from build123d import *

# Parameters (mm, degrees)
SKETCH1_R      = 2.5527
FINALCUT_DEPTH = 101.6


with BuildPart() as part:
    # Sketch1 → FinalCut (new body)
    with BuildSketch(Plane.XY):
        with BuildLine():
            Line((-17.4498, 0), (-17.4498, 3.187235435))
            Line((-17.4498, 3.187235435), (-23.0632, 8.800635435))
            Line((-23.0632, 8.800635435), (-23.0632, 3.2258))
            Line((-23.0632, 3.2258), (-25.4, 3.2258))
            Line((-25.4, 3.2258), (-25.4, 10.668))
            ThreePointArc((-25.4, 10.668), (-24.804840979, 12.104840979), (-23.368, 12.7))
            Line((-23.368, 12.7), (-15.9258, 12.7))
            Line((-15.9258, 12.7), (-15.9258, 10.3632))
            Line((-15.9258, 10.3632), (-21.500635435, 10.3632))
            Line((-21.500635435, 10.3632), (-15.887235435, 4.7498))
            Line((-15.887235435, 4.7498), (-12.7, 4.7498))
            Line((-12.7, 4.7498), (-9.512764565, 4.7498))
            Line((-9.512764565, 4.7498), (-3.899364565, 10.3632))
            Line((-3.899364565, 10.3632), (-9.4742, 10.3632))
            Line((-9.4742, 10.3632), (-9.4742, 12.7))
            Line((-9.4742, 12.7), (9.4742, 12.7))
            Line((9.4742, 12.7), (9.4742, 10.3632))
            Line((9.4742, 10.3632), (3.899364565, 10.3632))
            Line((3.899364565, 10.3632), (9.512764565, 4.7498))
            Line((9.512764565, 4.7498), (15.887235435, 4.7498))
            Line((15.887235435, 4.7498), (21.500635435, 10.3632))
            Line((21.500635435, 10.3632), (15.9258, 10.3632))
            Line((15.9258, 10.3632), (15.9258, 12.7))
            Line((15.9258, 12.7), (23.368, 12.7))
            ThreePointArc((23.368, 12.7), (24.804840979, 12.104840979), (25.4, 10.668))
            Line((25.4, 10.668), (25.4, 3.2258))
            Line((25.4, 3.2258), (23.0632, 3.2258))
            Line((23.0632, 3.2258), (23.0632, 8.800635435))
            Line((23.0632, 8.800635435), (17.4498, 3.187235435))
            Line((17.4498, 3.187235435), (17.4498, 0))
            Line((17.4498, 0), (17.4498, -3.187235435))
            Line((17.4498, -3.187235435), (23.0632, -8.800635435))
            Line((23.0632, -8.800635435), (23.0632, -3.2258))
            Line((23.0632, -3.2258), (25.4, -3.2258))
            Line((25.4, -3.2258), (25.4, -10.668))
            ThreePointArc((25.4, -10.668), (24.804840979, -12.104840979), (23.368, -12.7))
            Line((23.368, -12.7), (15.9258, -12.7))
            Line((15.9258, -12.7), (15.9258, -10.3632))
            Line((15.9258, -10.3632), (21.500635435, -10.3632))
            Line((21.500635435, -10.3632), (15.887235435, -4.7498))
            Line((15.887235435, -4.7498), (12.7, -4.7498))
            Line((12.7, -4.7498), (9.512764565, -4.7498))
            Line((9.512764565, -4.7498), (3.899364565, -10.3632))
            Line((3.899364565, -10.3632), (9.4742, -10.3632))
            Line((9.4742, -10.3632), (9.4742, -12.7))
            Line((9.4742, -12.7), (-9.4742, -12.7))
            Line((-9.4742, -12.7), (-9.4742, -10.3632))
            Line((-9.4742, -10.3632), (-3.899364565, -10.3632))
            Line((-3.899364565, -10.3632), (-9.512764565, -4.7498))
            Line((-9.512764565, -4.7498), (-12.7, -4.7498))
            Line((-12.7, -4.7498), (-15.887235435, -4.7498))
            Line((-15.887235435, -4.7498), (-21.500635435, -10.3632))
            Line((-21.500635435, -10.3632), (-15.9258, -10.3632))
            Line((-15.9258, -10.3632), (-15.9258, -12.7))
            Line((-15.9258, -12.7), (-23.368, -12.7))
            ThreePointArc((-23.368, -12.7), (-24.804840979, -12.104840979), (-25.4, -10.668))
            Line((-25.4, -10.668), (-25.4, -3.2258))
            Line((-25.4, -3.2258), (-23.0632, -3.2258))
            Line((-23.0632, -3.2258), (-23.0632, -8.800635435))
            Line((-23.0632, -8.800635435), (-17.4498, -3.187235435))
            Line((-17.4498, -3.187235435), (-17.4498, 0))
        make_face()
        with Locations((-12.7, 0)):
            Circle(SKETCH1_R, mode=Mode.SUBTRACT)
        with Locations(Location((12.7, 0, 0), (0, 0, 180))):
            Circle(SKETCH1_R, mode=Mode.SUBTRACT)
        Polygon((7.9502, 3.187235435), (0, 11.137435435), (-7.9502, 3.187235435), (-7.9502, 0), (-7.9502, -3.187235435), (0, -11.137435435), (7.9502, -3.187235435), (7.9502, 0), align=None, mode=Mode.SUBTRACT)
    extrude(amount=-FINALCUT_DEPTH)


solid = part.part
Work out the finished part from the listing and answer in its coordinate system (mm). A direction names the side the tool comes from. Give positions to 0.01 mm unless a question says otherwise; leave off trailing zeros. Write each loop counter-clockwise with the first axis right and the second up, starting at its lowest first coordinate (ties: lowest second). Pieces come first, ordered by that corner, then holes. Notation, with made-up numbers: (-4, -21) - (49, -21) arc R24 ccw to (49, -7) - close; hole circle Ø11 at (87, 43.5). An arc over 180 degrees is marked (long way). One line per item, written item: value. Start each with the question number.
1. Find section C-C (z = -85). State how many separate pieces and enclosed holes the cut face has, then the cut area to 3 significant figures.
2. Find section B-B (y = 0). Write down the section's boundary in (x, z), then the cut area to 3 significant figures.
3. Given pin 1 (5 mm diameter, centred on y = 3, z = -73, fed in from +X); pin 2 (1.2 mm diameter, centred on y = -11.5, z = -75, fed in from -X); pin 3 (3 mm diameter, centred on y = -0.5, z = -27.5, fed in from -X); pin 4 (3 mm diameter, centred on x = -14, z = -47.5, fed in from -Y), each flat-ended and moving along its own axis, determine where each tip first touches the part or whether it passes through.
4. For a pull along X with two mould halves and no side action, classify faces 5 (the cylindrical face through (-24.79, -12.12, -50.09)), 6 (the flat face through (6.745, -7.517, -50.089)), 7 (the flat face through (0, -12.7, -50)), 8 (the cylindrical face through (24.79, 12.12, -50.09)) as +X half, -X half, draft (parallel to the pull), parting line (faces both ways), or undercut.
5. Find section D-D (x = 20). Write down the section's boundary in (y, z), then the cut area to 3 significant figures.
6. Find section A-A (x = 12.7). Write down the section's boundary in (y, z).
7. Consider probe 1 along X at (y, z) = (0.25, -11); probe 2 along Y at (x, z) = (-12.7, -72); probe 3 along X at (y, z) = (10.75, -47). Determine where each line is inside the solid, lowest interval first.
8. For faces 1 (the flat face through (-24, 3.226, -50)), 2 (the flat face through (-15.926, 12, -50)), 3 (the flat face through (4.03, 7.11, -50.09)), 4 (the flat face through (15.926, -12, -50)), determine the directions among +Z, -Z, +X, -X, +Y, -Y from which every point of the face is accessible in a straight line to the end or side of a thin tool.
Geometry results:
1. separate pieces: 1
1. enclosed holes: 3
1. area: 524 mm2
2. outline: (-17.45, -101.6) - (-15.25, -101.6) - (-15.25, 0) - (-17.45, 0) - close; (-10.15, -101.6) - (-7.95, -101.6) - (-7.95, 0) - (-10.15, 0) - close; (7.95, -101.6) - (10.15, -101.6) - (10.15, 0) - (7.95, 0) - close; (15.25, -101.6) - (17.45, -101.6) - (17.45, 0) - (15.25, 0) - close
2. area: 893 mm2
3. pin 1: x = 25.4
3. pin 2: x = -25.39
3. pin 3: x = -17.45
3. pin 4: y = -4.75
4. face 5: -X half
4. face 6: undercut
4. face 7: draft
4. face 8: +X half
5. outline: (-12.7, -101.6) - (-10.36, -101.6) - (-10.36, 0) - (-12.7, 0) - close; (-8.86, -101.6) - (-5.74, -101.6) - (-5.74, 0) - (-8.86, 0) - close; (5.74, -101.6) - (8.86, -101.6) - (8.86, 0) - (5.74, 0) - close; (10.36, -101.6) - (12.7, -101.6) - (12.7, 0) - (10.36, 0) - close
5. area: 1,110 mm2
6. outline: (-4.75, -101.6) - (-2.55, -101.6) - (-2.55, 0) - (-4.75, 0) - close; (2.55, -101.6) - (4.75, -101.6) - (4.75, 0) - (2.55, 0) - close
7. probe 1: -17.45 to -15.24, -10.16 to -7.95, 7.95 to 10.16, 15.24 to 17.45
7. probe 2: -4.75 to -2.55, 2.55 to 4.75
7. probe 3: -25.4 to -15.93, -9.47 to -0.39, 0.39 to 9.47, 15.93 to 25.4
8. face 1: +Z, -Z, -X
8. face 2: +Z, -Z, +Y
8. face 3: +Z, -Z
8. face 4: +Z, -Z, -Y
